```python
from build123d import *

# Parameters (mm, degrees)
SKETCH_1_W                 = 20
SKETCH_1_H                 = 410
EXTRUDE_1_DEPTH            = 1.5
CUT_EXTRUDE_1_REACH        = 3.5
SKETCH_2_W                 = 3
SKETCH_2_H                 = 5
SKETCH_3_W                 = 20
SKETCH_3_H                 = 1.4
CUT_EXTRUDE_2_DEPTH        = 1.5
PATTERN_LINEAR_1_COUNT     = 6
PATTERN_LINEAR_1_PITCH     = 33.33
PATTERN_LINEAR_1_COL_COUNT = 6
PATTERN_LINEAR_1_COL_PITCH = 33.33


with BuildPart() as part:
    # 草图1 → 凸台-拉伸1 (new body)
    with BuildSketch(Plane.XY):
        Rectangle(SKETCH_1_W, SKETCH_1_H)
    extrude(amount=EXTRUDE_1_DEPTH)

    # 草图2 → 切除-拉伸1 (cut, up to next)
    with BuildSketch(Plane.XY.offset(1.5), mode=Mode.PRIVATE) as cut_extrude_1_sk1:
        with Locations((-8.5, 202.5)):
            Rectangle(SKETCH_2_W, SKETCH_2_H)
    cut_extrude_1_tool1 = extrude(cut_extrude_1_sk1.sketch, amount=-CUT_EXTRUDE_1_REACH, mode=Mode.PRIVATE) & part.part
    add(cut_extrude_1_tool1.solids().sort_by_distance((-8.5, 202.5, 1.5))[0], mode=Mode.SUBTRACT)
    # 草图2 → 切除-拉伸1 (cut, up to next)
    with BuildSketch(Plane.XY.offset(1.5), mode=Mode.PRIVATE) as cut_extrude_1_sk2:
        with Locations((8.5, 202.5)):
            Rectangle(SKETCH_2_W, SKETCH_2_H)
    cut_extrude_1_tool2 = extrude(cut_extrude_1_sk2.sketch, amount=-CUT_EXTRUDE_1_REACH, mode=Mode.PRIVATE) & part.part
    add(cut_extrude_1_tool2.solids().sort_by_distance((8.5, 202.5, 1.5))[0], mode=Mode.SUBTRACT)
    # 草图2 → 切除-拉伸1 (cut, up to next)
    with BuildSketch(Plane.XY.offset(1.5), mode=Mode.PRIVATE) as cut_extrude_1_sk3:
        with Locations((-8.5, -202.5)):
            Rectangle(SKETCH_2_W, SKETCH_2_H)
    cut_extrude_1_tool3 = extrude(cut_extrude_1_sk3.sketch, amount=-CUT_EXTRUDE_1_REACH, mode=Mode.PRIVATE) & part.part
    add(cut_extrude_1_tool3.solids().sort_by_distance((-8.5, -202.5, 1.5))[0], mode=Mode.SUBTRACT)
    # 草图2 → 切除-拉伸1 (cut, up to next)
    with BuildSketch(Plane.XY.offset(1.5), mode=Mode.PRIVATE) as cut_extrude_1_sk4:
        with Locations((8.5, -202.5)):
            Rectangle(SKETCH_2_W, SKETCH_2_H)
    cut_extrude_1_tool4 = extrude(cut_extrude_1_sk4.sketch, amount=-CUT_EXTRUDE_1_REACH, mode=Mode.PRIVATE) & part.part
    add(cut_extrude_1_tool4.solids().sort_by_distance((8.5, -202.5, 1.5))[0], mode=Mode.SUBTRACT)

    # 草图3 → 切除-拉伸2 (cut)
    with BuildSketch(Plane.XY.offset(1.5)):
        with Locations((-10, 0)):
            Rectangle(SKETCH_3_W, SKETCH_3_H)
    cut_extrude_2 = extrude(amount=-CUT_EXTRUDE_2_DEPTH, mode=Mode.SUBTRACT)

    # 阵列(线性)1: 切除-拉伸2 ×6
    with Locations(*[(0, i * PATTERN_LINEAR_1_PITCH, 0) for i in range(1, PATTERN_LINEAR_1_COUNT)]):
        add(cut_extrude_2, mode=Mode.SUBTRACT)

    # 阵列(线性)1 col: 切除-拉伸2 ×6
    with Locations(*[(0, -i * PATTERN_LINEAR_1_COL_PITCH, 0) for i in range(1, PATTERN_LINEAR_1_COL_COUNT)]):
        add(cut_extrude_2, mode=Mode.SUBTRACT)


solid = part.part
```
Geometry: final body of the model. Coordinates: model frame, mm. Round coordinates to 2 decimals unless told otherwise and drop trailing zeros. Use one line per item in the form item = value. Start each with the question number.
Q1. Cut plane A-A (x = -4). Count the separate pieces of the cut face and the enclosed holes in it, and give its area (3 significant figures).
Q2. Pin query (flat end, axial travel): pin 1 Ø0.8 at (y, z) = (202, 1) entering from +X. Return the tip coordinate at first contact, or that it passes through.
Q3. Material intervals for line 1 (Y direction, x = 8, z = 0.8), sorted ascending. Write a range as [from, to].
Geometry results:
q1.separate_pieces = 12
q1.enclosed_holes = 0
q1.area = 592 mm^2
q2.pin_1 = 7
q3.line_1 = [-200, 200]
